Geometry check sheet. Reference: the model listing, model coordinates, mm. Face numbers are marked on the shaded views. Coordinates: 2 decimals unless noted, no trailing zeros. Write each loop counter-clockwise with the first axis right and the second up, starting at its lowest first coordinate (ties: lowest second). Pieces come first, ordered by that corner, then holes. Notation, with made-up numbers: (-18, 45.5) -> (-12, 45.5) arc R17 cw to (-12, 70.5) -> close; hole circle Ø5 at (55, 22.5). An arc over 180 degrees is marked (long way). One line per question, with ' | ' between items.
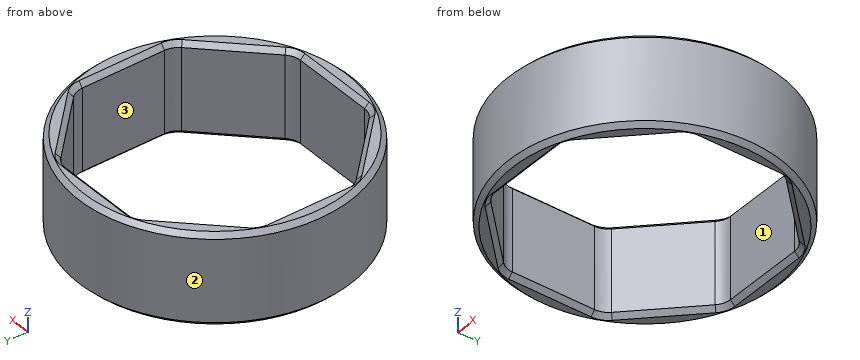
from build123d import *

# Parameters (mm, degrees)
SKETCH1_R           = 7.5
BOSS_EXTRUDE1_DEPTH = 2.5
FILLET1_R           = 1
CHAMFER1_SIZE       = 0.25


with BuildPart() as part:
    # Sketch1 → Boss-Extrude1 (new, symmetric)
    with BuildSketch(Plane.XY):
        Circle(SKETCH1_R)
        Polygon((-6.5, 2.692388155), (-6.5, -2.692388155), (-2.692388155, -6.5), (2.692388155, -6.5), (6.5, -2.692388155), (6.5, 2.692388155), (2.692388155, 6.5), (-2.692388155, 6.5), align=None, mode=Mode.SUBTRACT)
    extrude(amount=BOSS_EXTRUDE1_DEPTH, both=True)

    # Fillet1
    fillet1_edges = [part.edges().sort_by_distance(p)[0] for p in [
        (-6.5, -2.692388155, 0),
        (-6.5, 2.692388155, 0),
        (-2.692388155, -6.5, 0),
        (2.692388155, -6.5, 0),
        (6.5, -2.692388155, 0),
        (6.5, 2.692388155, 0),
        (2.692388155, 6.5, 0),
        (-2.692388155, 6.5, 0),
    ]]
    fillet(fillet1_edges, radius=FILLET1_R)

    # Chamfer1
    chamfer1_edges = [part.edges().sort_by_distance(p)[0] for p in [
        (-4.596194078, 4.596194078, 2.5),
        (-2.660858025, 6.423879533, 2.5),
        (-6.423879533, 2.660858025, 2.5),
        (0, 6.5, 2.5),
        (-6.5, 0, 2.5),
        (2.660858025, 6.423879533, 2.5),
        (-6.423879533, -2.660858025, 2.5),
        (4.596194078, 4.596194078, 2.5),
        (-4.596194078, -4.596194078, 2.5),
        (6.423879533, 2.660858025, 2.5),
        (-2.660858025, -6.423879533, 2.5),
        (6.5, 0, 2.5),
        (0, -6.5, 2.5),
        (6.423879533, -2.660858025, 2.5),
        (2.660858025, -6.423879533, 2.5),
        (4.596194078, -4.596194078, 2.5),
        (-7.5, 0, 2.5),
        (-4.596194078, 4.596194078, -2.5),
        (-2.660858025, 6.423879533, -2.5),
        (-6.423879533, 2.660858025, -2.5),
        (0, 6.5, -2.5),
        (-6.5, 0, -2.5),
        (2.660858025, 6.423879533, -2.5),
        (-6.423879533, -2.660858025, -2.5),
        (4.596194078, 4.596194078, -2.5),
        (-4.596194078, -4.596194078, -2.5),
        (6.423879533, 2.660858025, -2.5),
        (-2.660858025, -6.423879533, -2.5),
        (6.5, 0, -2.5),
        (0, -6.5, -2.5),
        (6.423879533, -2.660858025, -2.5),
        (2.660858025, -6.423879533, -2.5),
        (4.596194078, -4.596194078, -2.5),
        (-7.5, 0, -2.5),
    ]]
    chamfer(chamfer1_edges, length=CHAMFER1_SIZE)


solid = part.part
1. Go/stop test with flat-tipped pins: P1, Ø8, axis at x = -3.5, y = -4.5, coming from the -Z side; P2, Ø1.5, axis at y = 3.5, z = 1.5, coming from the +X side; P3, Ø1.5, axis at x = 3.5, z = -1.5, coming from the +Y side; P4, Ø2, axis at x = 5.5, z = -1, coming from the -Y side. Record where each tip stops, or that it passes through.
Worked answers:
P1: z = -2.5 | P2: x = 6.98 | P3: y = 6.98 | P4: y = -6
2. Cross-section at A-A on x = 0. Record the boundary of the cut face in (y, z).
Worked answers:
outline: (-7.5, -2.25) -> (-7.25, -2.5) -> (-6.75, -2.5) -> (-6.5, -2.25) -> (-6.5, 2.25) -> (-6.75, 2.5) -> (-7.25, 2.5) -> (-7.5, 2.25) -> close; (6.5, -2.25) -> (6.75, -2.5) -> (7.25, -2.5) -> (7.5, -2.25) -> (7.5, 2.25) -> (7.25, 2.5) -> (6.75, 2.5) -> (6.5, 2.25) -> close
3. Mould release check, pull along X, two halves, no side actions. Record for the marked faces 1, 2 and 3: released by +X, released by -X, zero draft, split by the parting line, or undercut.
Worked answers:
face 1: undercut | face 2: split by the parting line | face 3: undercut
4. Material ranges on line 1 (X direction, y = 0.25, z = -1.35); line 2 (Y direction, x = -4.75, z = -0.3); line 3 (X direction, y = -2.5, z = 1.75), recorded low to high. Write a range as from..to.
Worked answers:
line 1: -7.5..-6.5, 6.5..7.5 | line 2: -5.8..-4.44, 4.44..5.8 | line 3: -7.07..-6.48, 6.48..7.07
5. Cross-section at B-B on z = -0.3. Record the boundary of the cut face in (x, y).
Worked answers:
outline: circle Ø15 at (0, 0); hole (-6.5, -2.28) arc R1 ccw to (-6.21, -2.99) -> (-2.99, -6.21) arc R1 ccw to (-2.28, -6.5) -> (2.28, -6.5) arc R1 ccw to (2.99, -6.21) -> (6.21, -2.99) arc R1 ccw to (6.5, -2.28) -> (6.5, 2.28) arc R1 ccw to (6.21, 2.99) -> (2.99, 6.21) arc R1 ccw to (2.28, 6.5) -> (-2.28, 6.5) arc R1 ccw to (-2.99, 6.21) -> (-6.21, 2.99) arc R1 ccw to (-6.5, 2.28) -> close
